from build123d import *

# Parameters (mm, degrees)
SKETCH1_R           = 8
BOSS_EXTRUDE1_DEPTH = 5
SKETCH2_R           = 11
BOSS_EXTRUDE2_DEPTH = 4
SKETCH3_R           = 6
CUT_EXTRUDE1_DEPTH  = 18.972200756
BOSS_EXTRUDE3_START = -6
BOSS_EXTRUDE3_DEPTH = 0.25
SKETCH5_R           = 11
SKETCH5_R_2         = 10
CUT_EXTRUDE2_DEPTH  = 0.25
FILLET1_R           = 2


with BuildPart() as part:
    # Sketch1 → Boss-Extrude1 (new body)
    with BuildSketch(Plane(origin=(0, 0, 0), x_dir=(1, 0, 0), z_dir=(0, 1, 0))):
        with Locations(Location((0, 0, 0), (0, 0, 270))):
            Circle(SKETCH1_R)
    extrude(amount=BOSS_EXTRUDE1_DEPTH)

    # Sketch2 → Boss-Extrude2 (add)
    with BuildSketch(Plane(origin=(0, 5, 0), x_dir=(1, 0, 0), z_dir=(0, 1, 0))):
        with Locations(Location((0, 0, 0), (0, 0, 270))):
            Circle(SKETCH2_R)
    extrude(amount=BOSS_EXTRUDE2_DEPTH)

    # Sketch3 → Cut-Extrude1 (cut, through all)
    with BuildSketch(Plane(origin=(0, 9, 0), x_dir=(1, 0, 0), z_dir=(0, 1, 0))):
        with Locations(Location((0, 0, 0), (0, 0, 270))):
            Circle(SKETCH3_R)
    extrude(amount=-CUT_EXTRUDE1_DEPTH, mode=Mode.SUBTRACT)

    # Sketch4 → Boss-Extrude3 (add)
    with BuildSketch(Plane.XZ.offset(BOSS_EXTRUDE3_START)):
        with BuildLine():
            Line((0, 0.65), (-2.064316872, 5.633701789))
            ThreePointArc((-2.064316872, 5.633701789), (0, 6), (2.064316872, 5.633701789))
            Line((2.064316872, 5.633701789), (0, 0.65))
        make_face()
        with BuildLine():
            Line((0.562916512, 0.325), (3.846770431, 4.604601747))
            ThreePointArc((3.846770431, 4.604601747), (5.196152423, 3), (5.911087303, 1.029100042))
            Line((5.911087303, 1.029100042), (0.562916512, 0.325))
        make_face()
        with BuildLine():
            Line((0.562916512, -0.325), (5.911087303, -1.029100042))
            ThreePointArc((5.911087303, -1.029100042), (5.196152423, -3), (3.846770431, -4.604601747))
            Line((3.846770431, -4.604601747), (0.562916512, -0.325))
        make_face()
        with BuildLine():
            Line((0, -0.65), (2.064316872, -5.633701789))
            ThreePointArc((2.064316872, -5.633701789), (0, -6), (-2.064316872, -5.633701789))
            Line((-2.064316872, -5.633701789), (0, -0.65))
        make_face()
        with BuildLine():
            Line((-0.562916512, -0.325), (-3.846770431, -4.604601747))
            ThreePointArc((-3.846770431, -4.604601747), (-5.196152423, -3), (-5.911087303, -1.029100042))
            Line((-5.911087303, -1.029100042), (-0.562916512, -0.325))
        make_face()
        with BuildLine():
            Line((-0.562916512, 0.325), (-5.911087303, 1.029100042))
            ThreePointArc((-5.911087303, 1.029100042), (-5.196152423, 3), (-3.846770431, 4.604601747))
            Line((-3.846770431, 4.604601747), (-0.562916512, 0.325))
        make_face()
    extrude(amount=BOSS_EXTRUDE3_DEPTH)

    # Sketch5 → Cut-Extrude2 (cut)
    with BuildSketch(Plane.XZ.offset(-5)):
        with Locations(Location((0, 0, 0), (0, 0, 270))):
            Circle(SKETCH5_R)
        with Locations(Location((0, 0, 0), (0, 0, 270))):
            Circle(SKETCH5_R_2, mode=Mode.SUBTRACT)
    extrude(amount=-CUT_EXTRUDE2_DEPTH, mode=Mode.SUBTRACT)

    # Fillet1
    fillet1_edges = [part.edges().sort_by_distance(p)[0] for p in [
        (0, 9, -6),
        (0, 9, -11),
    ]]
    fillet(fillet1_edges, radius=FILLET1_R)


solid = part.part
Geometry check sheet. Reference: the model listing, model coordinates, mm. A direction names the side the tool comes from. Round coordinates to 2 decimals unless told otherwise and drop trailing zeros. Loops run counter-clockwise (first coordinate to the right, second up) from the corner with the lowest first, then second, coordinate; pieces in that order, holes last. Notation, with made-up numbers: (25.5, 83) -> (37.5, 83) arc R33 cw to (37.5, 113) -> close; hole circle Ø11 at (45.25, 31.25). An arc over 180 degrees is marked (long way). Answer as a JSON object with one key per item and string values. Group by question number.
Item 1: Cross-section at B-B, the plane y = 2.5. Record the cut outline in (x, z).
Item 2: Cross-section at A-A, the plane z = 0. Record the cut outline in (x, y).
Item 3: Cross-section at C-C, the plane x = 2.75. Count the separate pieces of the cut face and the enclosed holes in it, plus the area to 3 significant figures.
Item 4: Thickness scan on line 1 along X through (y, z) = (4.75, 0); line 2 along Y through (x, z) = (7.75, 3); line 3 along Y through (x, z) = (-0.75, -3.75). Record the ranges inside material, lowest first.
Item 5: Depth check by flat-ended pin: pin 1 Ø3.5 at (x, z) = (-4.5, -3) entering from +Y; pin 2 Ø2 at (x, z) = (2.5, -2) entering from -Y; pin 3 Ø1.3 at (x, z) = (3.5, -2) entering from +Y. Enter the tip coordinate at first touch or a pass-through.
Item 6: Release check for a two-part mould opening along Z. For faces 1 (the face through (-7.81, 2.46, -1.73)), 2 (the face through (0, 5.75, 4)), 3 (the face through (-10, 5.25, -2)), 4 (the face through (4, 5.75, -2)) record: pulls with the +Z half, pulls with the -Z half, needs draft (parallel to the pull), parting line crosses it, or undercut.
Item 7: Set-up check for faces 5 (the face through (4, 5.75, 2)), 6 (the face through (-10.74, 6.11, -2.38)), 7 (the face through (0, 6, -4)): record each of +Z, -Z, +X, -X, +Y, -Y from which the full face is reachable in a straight line by a thin tool's end or side.
Determined:
{
 "1": {"outline": "circle Ø16 at (0, 0); hole circle Ø12 at (0, 0)"},
 "2": {"outline": "(-11, 5.25) -> (-10, 5.25) -> (-10, 5) -> (-8, 5) -> (-8, 0) -> (-6, 0) -> (-6, 7) arc R2 ccw to (-8, 9) -> (-9, 9) arc R2 ccw to (-11, 7) -> close; (6, 0) -> (8, 0) -> (8, 5) -> (10, 5) -> (10, 5.25) -> (11, 5.25) -> (11, 7) arc R2 ccw to (9, 9) -> (8, 9) arc R2 ccw to (6, 7) -> close"},
 "3": {"separate pieces": "4", "enclosed holes": "0", "area": "61.4 mm²"},
 "4": {"line 1": "x = -8 to -6, 6 to 8", "line 2": "y = 5 to 9", "line 3": "y = 5.75 to 6"},
 "5": {"pin 1": "stops at y = 8.81", "pin 2": "stops at y = 5.75", "pin 3": "stops at y = 6"},
 "6": {"face 1": "parting line crosses it", "face 2": "undercut", "face 3": "needs draft", "face 4": "undercut"},
 "7": {"face 5": "-Y", "face 6": "+Y, -Y", "face 7": "+Y"}
}
